Solid Edge part; units mm, degrees
sketch "Sketch1" plane through (0, 0, 0) normal (0, -1, 0) x (1, 0, 0)
  arc A0 (-37.1299, 86.2147) -> (92.6101, -40.7853) centre (-39.0034, -45.4688) cw
  line L0 (92.6101, -40.7853) -> (92.6101, -101.2453)
  line L1 (92.6101, -101.2453) -> (95.6101, -101.2453)
  line L2 (95.6101, -101.2453) -> (95.6101, -40.7853)
  arc A1 (-37.1299, 89.2147) -> (95.6101, -40.7853) centre (-39.0019, -45.4657) cw
  line L3 (-97.1299, 89.2147) -> (-37.1299, 89.2147)
  line L4 (-97.1299, 86.2147) -> (-97.1299, 89.2147)
  line L5 (-37.1299, 86.2147) -> (-97.1299, 86.2147)
  dimension "D1" = 37.1299
  dimension "D2" = 92.6101
  dimension "D3" = 37.1299
  dimension "D4" = 95.6101
extrude "Protrusion1" add sketch "Sketch1" against normal blind 204
sketch "Sketch2" plane through (-67.1299, 85, 89.2147) normal (0, 0, 1) x (1, 0, 0)
  circle A0 centre (-6.3, -58.5) radius 2.25
  circle A1 centre (-6.3, 56.5) radius 2.25
  dimension "D1" = 6.3
extrude "Cutout1" cut sketch "Sketch2" against normal through all
sketch "Sketch3" plane through (95.6101, 85, -66.0153) normal (1, 0, 0) x (0, 1, 0)
  circle A0 centre (58, -11.65) radius 2.25
  circle A1 centre (-56, -11.65) radius 2.25
  dimension "D1" = 56
  dimension "D2" = 56
extrude "Cutout2" cut sketch "Sketch3" against normal through all
sketch "Sketch4" plane through (-97.1299, 102, 87.7147) normal (-1, 0, 0) x (0, -1, 0)
  line L0 (-102, -1.5) -> (102, -1.5)
  line L1 (102, -1.5) -> (102, 1.5)
  line L2 (102, 1.5) -> (-102, 1.5)
  line L3 (-102, 1.5) -> (-102, -1.5)
extrude "Extrusionsausprägung_3" add sketch "Sketch4" along normal blind 1.3
sketch "Sketch5" plane through (94.1101, 102, -101.2453) normal (0, 0, -1) x (0, 1, 0)
  line L0 (-102, 1.5) -> (102, 1.5)
  line L1 (102, 1.5) -> (102, -1.5)
  line L2 (102, -1.5) -> (-102, -1.5)
  line L3 (-102, -1.5) -> (-102, 1.5)
extrude "Extrusionsausprägung_4" add sketch "Sketch5" along normal blind 1.42
sketch "Sketch6" plane through (-67.7799, 102, 89.2147) normal (0, 0, 1) x (0, 1, 0)
  line L0 (21.17, 30.65) -> (-14.2216, -30.65)
  line L1 (-14.2216, -30.65) -> (-28.6553, -30.65)
  line L2 (-28.6553, -30.65) -> (6.7362, 30.65)
  line L3 (6.7362, 30.65) -> (21.17, 30.65)
  dimension "D1" = 21.17
extrude "Extrusionsausschnitt_3" cut sketch "Sketch6" against normal blind 1
chamfer "Fase_1" distance 0.5 angle 60 4 edges at (-75.6799, 26.5, 89.2147) (-75.6799, 141.5, 89.2147) (95.6101, 26.75, -77.6653) (95.6101, 140.75, -77.6653) measured on face at (-87.7299, 88.9082, 89.2147) measured on face at (-87.7299, 183.4675, 89.2147) measured on face at (-87.7299, 88.9082, 89.2147) measured on face at (-87.7299, 183.4675, 89.2147) measured on face at (95.6101, 167.96, -91.7732)
sketch "Sketch7" plane through (-67.7799, 145.8892, 89.2147) normal (0, 0, 1) x (-1, 0, 0)
  line L0 (30.65, -58.1108) -> (-160.39, -58.1108)
  line L1 (-160.39, -58.1108) -> (-160.39, -53.1108)
  line L2 (-160.39, -53.1108) -> (30.65, -53.1108)
  line L3 (30.65, -53.1108) -> (30.65, -58.1108)
  dimension "D1" = 30.65
  dimension "D2" = 30.65
extrude "Cutout3" cut sketch "Sketch7" against normal up to next
sketch "Sketch8" plane through (94.1101, 204, -59.7426) normal (0, 1, 0) x (0, 0, -1)
  line L0 (-42.9227, 1.5) -> (42.9227, 1.5)
  line L1 (42.9227, 1.5) -> (42.9227, -1.5)
  line L2 (42.9227, -1.5) -> (-18.9573, -1.5)
  arc A0 (-18.9573, -1.5) -> (-42.9227, 1.5) centre (-14.2769, 133.1121) cw
extrude "Extrusionsausprägung_7" add sketch "Sketch8" along normal blind 3
sketch "Sketch9" plane through (92.6101, 103.5, -59.7426) normal (-1, 0, 0) x (0, -1, 0)
  line L0 (-88.5, 42.9227) -> (-93.5, 42.9227)
  line L1 (-93.5, 42.9227) -> (-93.5, -42.9227)
  line L2 (-93.5, -42.9227) -> (-88.5, -42.9227)
  line L3 (-88.5, -42.9227) -> (-88.5, 42.9227)
  line L4 (-103.5, 42.9227) -> (-100.5, 42.9227)
  line L5 (-100.5, 42.9227) -> (-100.5, -42.9227)
  line L6 (-100.5, -42.9227) -> (-103.5, -42.9227)
  line L7 (-103.5, -42.9227) -> (-103.5, 42.9227)
  dimension "D1" = 100.5
  dimension "D2" = 93.5
  dimension "D3" = 88.5
extrude "Extrusionsausprägung_8" add sketch "Sketch9" along normal blind 20
sketch "Sketch10" plane through (84.1101, 103.5, -102.6653) normal (0, 0, -1) x (0, 1, 0)
  line L0 (93.5, 8.5) -> (93.5, -182.54)
  line L1 (93.5, -182.54) -> (97, -182.54)
  line L2 (97, -182.54) -> (97, 8.5)
  line L3 (97, 8.5) -> (93.5, 8.5)
extrude "Cutout4" cut sketch "Sketch10" against normal up to next
properties material "Nylon, allgemein"
Check sheet for the modelled part. Datum: model origin and axes. Units: mm. A direction names the side the tool comes from. Round coordinates to 2 decimals unless told otherwise and drop trailing zeros. Write each loop counter-clockwise with the first axis right and the second up, starting at its lowest first coordinate (ties: lowest second). Pieces come first, ordered by that corner, then holes. Notation, with made-up numbers: (25.25, 60.25) -> (31.25, 60.25) arc R28 ccw to (31.25, 89.25) -> close; hole circle Ø9 at (76, -36). An arc over 180 degrees is marked (long way). One line per question, with ' | ' between items. Start each with the question number.
1. Scan lines: line 1 along Z through (x, y) = (-47, 28); line 2 along X through (y, z) = (139, -87); line 3 along Z through (x, y) = (82, 71.5). Record each from-to range of solid material in increasing order. Write a range as from..to.
2. Depth check by flat-ended pin: pin 1 (1.5 mm diameter, centred on x = 85.5, y = 205.5, fed in from +Z); pin 2 (6 mm diameter, centred on y = 185.5, z = 8, fed in from +X); pin 3 (0.7 mm diameter, centred on y = 87.5, z = -102, fed in from -X); pin 4 (4 mm diameter, centred on x = -73.43, y = 141.5, fed in from -Z). Enter the tip coordinate at first touch or a pass-through.
3. Sectioned sample at C-C, the plane x = -40.5. Record the cut outline in (y, z).
4. Release check for a two-part mould opening along Y. For faces 5 (the face through (-68.209, 105.722, 88.722)), 6 (the face through (93, 127, -102.665)), 7 (the face through (84, 207, -59)), 8 (the face through (83, 204, -59)) record: +Y half, -Y half, draft (parallel to the pull), parting line (faces both ways), or undercut.
5. Set-up check for faces 1 (the face through (56.26, 100.57, 49.76)), 2 (the face through (75, 197, -36)), 3 (the face through (-67.35, 90.79, 88.72)), 4 (the face through (83, 192, -60)): record each of +Z, -Z, +X, -X, +Y, -Y from which the full face is reachable in a straight line by a thin tool's end or side.
6. Sectioned sample at A-A, the plane y = 163.5. Record the cut outline in (x, z).
7. Sectioned sample at B-B, the plane z = -60.5. Record the cut outline in (x, y).
8. Sectioned sample at D-D, the plane y = 119. Record the cut outline in (x, z).
Taken from the geometry:
1) line 1: z = 86.21..89.21 | line 2: x = 92.61..95.61 | line 3: z = 6.51..13.7
2) pin 1: stops at z = -16.82 | pin 2: stops at x = 85.88 | pin 3: stops at x = 92.61 | pin 4: passes through
3) outline: (0, 86.21) -> (197, 86.21) -> (197, 89.21) -> (89.72, 89.21) -> (89.72, 88.21) -> (75.29, 88.21) -> (75.29, 89.21) -> (0, 89.21) -> close
4) face 5: undercut | face 6: draft | face 7: +Y half | face 8: undercut
5) face 1: +Z, +X, +Y, -Y | face 2: +Z, -Z, -X | face 3: +Z | face 4: -Z, -X, -Y
6) outline: (-98.43, 86.21) -> (-97.13, 86.21) -> (-37.13, 86.21) arc R131.7 cw to (92.61, -40.79) -> (92.61, -101.25) -> (92.61, -102.67) -> (95.61, -102.67) -> (95.61, -101.25) -> (95.61, -40.79) arc R134.69 ccw to (-37.13, 89.21) -> (-97.13, 89.21) -> (-98.43, 89.21) -> close
7) outline: (72.61, 192) -> (92.61, 192) -> (92.61, 0) -> (95.61, 0) -> (95.61, 207) -> (72.61, 207) -> (72.61, 204) -> (92.61, 204) -> (92.61, 197) -> (72.61, 197) -> close
8) outline: (-98.43, 86.21) -> (-97.13, 86.21) -> (-37.13, 86.21) arc R131.7 cw to (92.61, -40.79) -> (92.61, -101.25) -> (92.61, -102.67) -> (95.61, -102.67) -> (95.61, -101.25) -> (95.61, -40.79) arc R134.69 ccw to (-37.13, 89.21) -> (-91.21, 89.21) -> (-91.21, 88.21) -> (-98.43, 88.21) -> close
